from build123d import *

# Parameters (mm, degrees)
SKICA1_W                = 3
SKICA1_H                = 3
SKICA1_R                = 1
SKICA1_H_2              = 147
P_IDAT_VYSUNUT_M1_DEPTH = 3
P_IDAT_VYSUNUT_M3_DEPTH = 3


with BuildPart() as part:
    # Skica1 → Přidat vysunutím1 (new body)
    # profile 1 of 5: a face of its own
    with BuildSketch(Plane.XY):
        with Locations((4.5, 151.5)):
            Rectangle(SKICA1_W, SKICA1_H)
        with Locations((4.5, 151.5)):
            Circle(SKICA1_R, mode=Mode.SUBTRACT)
    # profile 2 of 5: a face of its own
    with BuildSketch(Plane.XY):
        with Locations((1.5, 151.5)):
            Rectangle(SKICA1_W, SKICA1_H)
    # profile 3 of 5: a face of its own
    with BuildSketch(Plane.XY):
        with Locations((1.5, 76.5)):
            Rectangle(SKICA1_W, SKICA1_H_2)
    # profile 4 of 5: a face of its own
    with BuildSketch(Plane.XY):
        with Locations((1.5, 1.5)):
            Rectangle(SKICA1_W, SKICA1_H)
    # profile 5 of 5: a face of its own
    with BuildSketch(Plane.XY):
        with Locations((4.5, 1.5)):
            Rectangle(SKICA1_W, SKICA1_H)
        with Locations((4.5, 1.5)):
            Circle(SKICA1_R, mode=Mode.SUBTRACT)
    extrude(amount=P_IDAT_VYSUNUT_M1_DEPTH)

    # Skica6 → Přidat vysunutím3 (add)
    with BuildSketch(Plane.ZY):
        Polygon((150, 3), (3, 153), (3, 148.713848419), (145.79957145, 3), (3, 3), (3, 0), (150, 0), align=None)
    extrude(amount=-P_IDAT_VYSUNUT_M3_DEPTH)


solid = part.part
Could you check a few things on this model? Use its own coordinates, in mm. Round coordinates to 2 decimals unless told otherwise and drop trailing zeros. Order: outer loops, then holes, each group sorted by start corner. A loop starts at its lowest first (then second) coordinate and runs counter-clockwise, first axis right, second up.
(1) Imagine slicing it at A-A (x = 4.5). Write out the boundary of the cut face in (y, z).
Response values:
outline: (0, 0) - (0.5, 0) - (0.5, 3) - (0, 3) - close; (2.5, 0) - (3, 0) - (3, 3) - (2.5, 3) - close; (150, 0) - (150.5, 0) - (150.5, 3) - (150, 3) - close; (152.5, 0) - (153, 0) - (153, 3) - (152.5, 3) - close
(2) If we mould it in two halves opening along Y, with no side actions, what happens to faces 1 (the flat face through (1.48, 76.95, 77.53)), 2 (the flat face through (2, 78, 0)), 3 (the flat face through (3, 94, 58)), 4 (the flat face through (1.479, 76.877, 73.4))? For each: released by +Y, released by -Y, zero draft, split by the parting line, or undercut.
Response values:
face 1: released by +Y
face 2: zero draft
face 3: undercut
face 4: undercut
(3) I'm going to push flat-ended pins straight in: pin 1 (1.5 mm diameter, centred on x = 4.5, y = 152, fed in from +Z); pin 2 (1.5 mm diameter, centred on x = 1.5, z = 92, fed in from +Y); pin 3 (3.5 mm diameter, centred on x = 1, y = 99, fed in from +Z) (3 decimals). Where does each tip first touch, or does it pass through?
Response values:
pin 1: stops at z = 3
pin 2: stops at y = 62.95
pin 3: stops at z = 57.635
(4) Please list where these lines run through material, in increasing order: line 1 along Y through (x, z) = (4.5, 2.2); line 2 along X through (y, z) = (151.5, 0.9); line 3 along Z through (x, y) = (1.75, 29).
Response values:
line 1: y = 0 to 0.5, 2.5 to 3, 150 to 150.5, 152.5 to 153
line 2: x = 0 to 3.5, 5.5 to 6
line 3: z = 0 to 3, 120.32 to 124.52
(5) Imagine slicing it at C-C (z = 48.5). Write out the boundary of the cut face in (x, y), plus the area to 3 significant figures.
Response values:
outline: (0, 0) - (3, 0) - (3, 3) - (0, 3) - close; (0, 102.29) - (3, 102.29) - (3, 106.57) - (0, 106.57) - close
area: 21.9 mm2
(6) Imagine slicing it at B-B (y = 121.5). Write out the boundary of the cut face in (x, z), plus the area to 3 significant figures.
Response values:
outline: (0, 0) - (3, 0) - (3, 3) - (0, 3) - close; (0, 29.67) - (3, 29.67) - (3, 33.87) - (0, 33.87) - close
area: 21.6 mm2
